Check sheet for the modelled part. Datum: model origin and axes. Units: mm. A direction names the side the tool comes from. Coordinates: 2 decimals unless noted, no trailing zeros. Write each loop counter-clockwise with the first axis right and the second up, starting at its lowest first coordinate (ties: lowest second). Pieces come first, ordered by that corner, then holes. Notation, with made-up numbers: M 1,39.25 L 7,39.25 A10 ccw 7,56.25 Z; hole C 22,84.25 d9. An arc over 180 degrees is marked long. Answer as CSV lines item,"result". Start each with the question number.
Q1. Sectioned sample at D-D, the plane z = 3.75. Record the cut outline in (x, y), then the cut area to 3 significant figures.
Q2. Mould release check, pull along X, two halves, no side actions. Record for faces 4 (the cylindrical face through (2.744, -3.517, 2.771)), 5 (the flat face through (-1.4, -4.5, -4.2)), 6 (the cylindrical face through (2.42, -4.36, 2.39)), 7 (the cylindrical face through (-2.42, -4.36, -2.39)): pulls with the +X half, pulls with the -X half, needs draft (parallel to the pull), parting line crosses it, or undercut.
Q3. Sectioned sample at B-B, the plane y = -3.3. Count the separate pieces of the cut face and the enclosed holes in it, then the cut area to 3 significant figures.
Q4. Sectioned sample at C-C, the plane z = 0. Record the cut outline in (x, y) (3 decimals).
Q5. Access from +Z, -Z, +X, -X, +Y, -Y to the whole of each face (thin tool, end or side, straight path). Record for faces 1 (the cylindrical face through (4.725, -4.192, 0.02)), 2 (the cylindrical face through (0, -4.3, 4.4)), 3 (the cylindrical face through (2.48, -2.96, 2.47)).
Q6. Depth check by flat-ended pin: pin 1 Ø0.6 at (x, y) = (-5, -4.5) entering from -Z; pin 2 Ø1.2 at (y, z) = (-4.5, 4.5) entering from -X; pin 3 Ø0.6 at (x, z) = (0.5, -4.5) entering from +Y. Enter the tip coordinate at first touch or a pass-through.
Q7. Sectioned sample at A-A, the plane x = 0. Record the cut outline in (y, z) (3 decimals).
Q8. Thickness scan on line 1 along Z through (x, y) = (-1, -3.95); line 2 along X through (y, z) = (-4.15, -3); line 3 along X through (y, z) = (-4.15, 2). Record the ranges inside material, lowest first. Write a range as from..to.
from build123d import *

# Parameters (mm, degrees)
SKETCH_1_R          = 3.4
EXTRUDE_1_DEPTH     = 1.1
EXTRUDE_START       = -0.362295
EXTRUDE_2_DEPTH     = 1.1
EXTRUDE_START_2     = -1.1
EXTRUDE_3_DEPTH     = 0.3
EXTRUDE_START_3     = 1.1
EXTRUDE_4_DEPTH     = 1.7
FILLET_2_R          = 0.5
FILLET_3_R          = 0.4
CUT_EXTRUDE_1_DEPTH = 8.685701009
FILLET_5_R          = 0.4


with BuildPart() as part:
    # 草图1 → 凸台-拉伸1 (new body)
    with BuildSketch(Plane.XZ.offset(4.897705057)):
        with BuildLine():
            Line((1.4, 4.38178046), (1.4, 3.640054945))
            ThreePointArc((1.4, 3.640054945), (2.757716447, 2.757716447), (3.640054945, 1.4))
            Line((3.640054945, 1.4), (4.38178046, 1.4))
            ThreePointArc((4.38178046, 1.4), (4.6, 0), (4.38178046, -1.4))
            Line((4.38178046, -1.4), (3.640054945, -1.4))
            ThreePointArc((3.640054945, -1.4), (2.757716447, -2.757716447), (1.4, -3.640054945))
            Line((1.4, -3.640054945), (1.4, -4.38178046))
            ThreePointArc((1.4, -4.38178046), (0, -4.6), (-1.4, -4.38178046))
            Line((-1.4, -4.38178046), (-1.4, -3.640054945))
            ThreePointArc((-1.4, -3.640054945), (-2.757716447, -2.757716447), (-3.640054945, -1.4))
            Line((-3.640054945, -1.4), (-4.38178046, -1.4))
            ThreePointArc((-4.38178046, -1.4), (-4.6, 0), (-4.38178046, 1.4))
            Line((-4.38178046, 1.4), (-3.640054945, 1.4))
            ThreePointArc((-3.640054945, 1.4), (-2.757716447, 2.757716447), (-1.4, 3.640054945))
            Line((-1.4, 3.640054945), (-1.4, 4.38178046))
            ThreePointArc((-1.4, 4.38178046), (0, 4.6), (1.4, 4.38178046))
        make_face()
        with Locations(Location((0, 0, 0), (0, 0, 270))):
            Circle(SKETCH_1_R, mode=Mode.SUBTRACT)
    extrude(amount=-EXTRUDE_1_DEPTH)

    # 草图2 → 凸台-拉伸2 (add)
    with BuildSketch(Plane.XZ.offset(4.16).offset(EXTRUDE_START)):
        with BuildLine():
            Line((4.276680956, 1.4), (4.512828935, 1.4))
            ThreePointArc((4.512828935, 1.4), (4.725, 0), (4.512828935, -1.4))
            Line((4.512828935, -1.4), (4.276680956, -1.4))
            ThreePointArc((4.276680956, -1.4), (4.5, 0), (4.276680956, 1.4))
        make_face()
        with BuildLine():
            Line((1.4, -4.276680956), (1.4, -4.512828935))
            ThreePointArc((1.4, -4.512828935), (0, -4.725), (-1.4, -4.512828935))
            Line((-1.4, -4.512828935), (-1.4, -4.276680956))
            ThreePointArc((-1.4, -4.276680956), (0, -4.5), (1.4, -4.276680956))
        make_face()
        with BuildLine():
            Line((-4.276680956, -1.4), (-4.512828935, -1.4))
            ThreePointArc((-4.512828935, -1.4), (-4.725, 0), (-4.512828935, 1.4))
            Line((-4.512828935, 1.4), (-4.276680956, 1.4))
            ThreePointArc((-4.276680956, 1.4), (-4.5, 0), (-4.276680956, -1.4))
        make_face()
        with BuildLine():
            Line((-1.4, 4.276680956), (-1.4, 4.512828935))
            ThreePointArc((-1.4, 4.512828935), (0, 4.725), (1.4, 4.512828935))
            Line((1.4, 4.512828935), (1.4, 4.276680956))
            ThreePointArc((1.4, 4.276680956), (0, 4.5), (-1.4, 4.276680956))
        make_face()
    extrude(amount=EXTRUDE_2_DEPTH)

    # 草图3 → 凸台-拉伸3 (add)
    with BuildSketch(Plane(origin=(0, -3.797705057, 0), x_dir=(-1, 0, 0), z_dir=(0, 1, 0)).offset(EXTRUDE_START_2)):
        with BuildLine():
            Line((4.276680956, 1.4), (5.111751168, 1.4))
            ThreePointArc((5.111751168, 1.4), (5.3, 0), (5.111751168, -1.4))
            Line((5.111751168, -1.4), (4.276680956, -1.4))
            ThreePointArc((4.276680956, -1.4), (4.5, 0), (4.276680956, 1.4))
        make_face()
        with BuildLine():
            Line((-1.4, -4.276680956), (-1.4, -5.111751168))
            ThreePointArc((-1.4, -5.111751168), (0, -5.3), (1.4, -5.111751168))
            Line((1.4, -5.111751168), (1.4, -4.276680956))
            ThreePointArc((1.4, -4.276680956), (0, -4.5), (-1.4, -4.276680956))
        make_face()
        with BuildLine():
            Line((-4.276680956, 1.4), (-5.111751168, 1.4))
            ThreePointArc((-5.111751168, 1.4), (-5.3, 0), (-5.111751168, -1.4))
            Line((-5.111751168, -1.4), (-4.276680956, -1.4))
            ThreePointArc((-4.276680956, -1.4), (-4.5, 0), (-4.276680956, 1.4))
        make_face()
        with BuildLine():
            Line((1.4, 4.276680956), (1.4, 5.111751168))
            ThreePointArc((1.4, 5.111751168), (0, 5.3), (-1.4, 5.111751168))
            Line((-1.4, 5.111751168), (-1.4, 4.276680956))
            ThreePointArc((-1.4, 4.276680956), (0, 4.5), (1.4, 4.276680956))
        make_face()
    extrude(amount=EXTRUDE_3_DEPTH)

    # 草图4 → 凸台-拉伸4 (add)
    with BuildSketch(Plane(origin=(0, -4.897705057, 0), x_dir=(-1, 0, 0), z_dir=(0, 1, 0)).offset(EXTRUDE_START_3)):
        with BuildLine():
            Line((1.55, 3.578756767), (1.55, 3.138072657))
            ThreePointArc((1.55, 3.138072657), (2.474873734, 2.474873734), (3.138072657, 1.55))
            Line((3.138072657, 1.55), (3.578756767, 1.55))
            ThreePointArc((3.578756767, 1.55), (2.757716447, 2.757716447), (1.55, 3.578756767))
        make_face()
        with BuildLine():
            Line((1.55, -3.138072657), (1.55, -3.578756767))
            ThreePointArc((1.55, -3.578756767), (2.757716447, -2.757716447), (3.578756767, -1.55))
            Line((3.578756767, -1.55), (3.138072657, -1.55))
            ThreePointArc((3.138072657, -1.55), (2.474873734, -2.474873734), (1.55, -3.138072657))
        make_face()
        with BuildLine():
            Line((-3.138072657, -1.55), (-3.578756767, -1.55))
            ThreePointArc((-3.578756767, -1.55), (-2.757716447, -2.757716447), (-1.55, -3.578756767))
            Line((-1.55, -3.578756767), (-1.55, -3.138072657))
            ThreePointArc((-1.55, -3.138072657), (-2.474873734, -2.474873734), (-3.138072657, -1.55))
        make_face()
        with BuildLine():
            Line((-1.55, 3.138072657), (-1.55, 3.578756767))
            ThreePointArc((-1.55, 3.578756767), (-2.757716447, 2.757716447), (-3.578756767, 1.55))
            Line((-3.578756767, 1.55), (-3.138072657, 1.55))
            ThreePointArc((-3.138072657, 1.55), (-2.474873734, 2.474873734), (-1.55, 3.138072657))
        make_face()
    extrude(amount=EXTRUDE_4_DEPTH)

    # 圆角2
    fillet_2_edges = [part.edges().sort_by_distance(p)[0] for p in [
        (1.55, -2.947705057, 3.138072657),
        (3.138072657, -2.947705057, 1.55),
        (3.138072657, -2.947705057, -1.55),
        (1.55, -2.947705057, -3.138072657),
        (-1.55, -2.947705057, -3.138072657),
        (-3.138072657, -2.947705057, -1.55),
        (-3.138072657, -2.947705057, 1.55),
        (-1.55, -2.947705057, 3.138072657),
    ]]
    fillet(fillet_2_edges, radius=FILLET_2_R)

    # 圆角3
    fillet_3_edges = [part.edges().sort_by_distance(p)[0] for p in [
        (-3.640054945, -4.347705057, 1.4),
        (-3.640054945, -4.347705057, -1.4),
        (-1.4, -4.347705057, -3.640054945),
        (1.4, -4.347705057, -3.640054945),
        (3.640054945, -4.347705057, -1.4),
        (3.640054945, -4.347705057, 1.4),
        (1.4, -4.347705057, 3.640054945),
        (-1.4, -4.347705057, 3.640054945),
    ]]
    fillet(fillet_3_edges, radius=FILLET_3_R)

    # 草图5 → 切除-拉伸1 (cut, through all)
    with BuildSketch(Plane(origin=(0, -3.797705057, 0), x_dir=(-1, 0, 0), z_dir=(0, 1, 0))):
        with BuildLine():
            Line((4.306971093, 0.9), (2.740001738, 0.9))
            Line((2.740001738, 0.9), (2.740001738, -0.9))
            Line((2.740001738, -0.9), (4.306971093, -0.9))
            ThreePointArc((4.306971093, -0.9), (4.4, 0), (4.306971093, 0.9))
        make_face()
        with BuildLine():
            Line((0.9, -4.306971093), (0.9, -2.740001738))
            Line((0.9, -2.740001738), (-0.9, -2.740001738))
            Line((-0.9, -2.740001738), (-0.9, -4.306971093))
            ThreePointArc((-0.9, -4.306971093), (0, -4.4), (0.9, -4.306971093))
        make_face()
        with BuildLine():
            Line((-4.306971093, -0.9), (-2.740001738, -0.9))
            Line((-2.740001738, -0.9), (-2.740001738, 0.9))
            Line((-2.740001738, 0.9), (-4.306971093, 0.9))
            ThreePointArc((-4.306971093, 0.9), (-4.4, 0), (-4.306971093, -0.9))
        make_face()
        with BuildLine():
            Line((-0.9, 4.306971093), (-0.9, 2.740001738))
            Line((-0.9, 2.740001738), (0.9, 2.740001738))
            Line((0.9, 2.740001738), (0.9, 4.306971093))
            ThreePointArc((0.9, 4.306971093), (0, 4.4), (-0.9, 4.306971093))
        make_face()
    extrude(amount=-CUT_EXTRUDE_1_DEPTH, mode=Mode.SUBTRACT)

    # 圆角5
    fillet_5_edges = [part.edges().sort_by_distance(p)[0] for p in [
        (0.9, -4.347705057, 3.278719262),
        (-0.9, -4.347705057, 3.278719262),
        (3.278719262, -4.347705057, -0.9),
        (3.278719262, -4.347705057, 0.9),
        (-0.9, -4.347705057, -3.278719262),
        (0.9, -4.347705057, -3.278719262),
        (-3.278719262, -4.347705057, 0.9),
        (-3.278719262, -4.347705057, -0.9),
        (-4.306971093, -4.347705057, -0.9),
        (-4.306971093, -4.347705057, 0.9),
        (0.9, -4.347705057, -4.306971093),
        (-0.9, -4.347705057, -4.306971093),
        (4.306971093, -4.347705057, 0.9),
        (4.306971093, -4.347705057, -0.9),
        (-0.9, -4.347705057, 4.306971093),
        (0.9, -4.347705057, 4.306971093),
    ]]
    fillet(fillet_5_edges, radius=FILLET_5_R)


solid = part.part
Output:
1,outline,"M -1.43,-4.9 L -0.9,-4.9 L -0.9,-3.8 L -1.43,-3.8 Z; M 0.9,-4.9 L 1.43,-4.9 L 1.43,-3.8 L 0.9,-3.8 Z"
1,area,"1.17 mm^2"
2,face 4,"pulls with the +X half"
2,face 5,"pulls with the -X half"
2,face 6,"undercut"
2,face 7,"undercut"
3,separate pieces,"4"
3,enclosed holes,"0"
3,area,"4.07 mm^2"
4,outline,"M -5.3,-4.898 L -4.4,-4.898 L -4.4,-3.798 L -4.725,-3.798 L -4.725,-4.598 L -5.3,-4.598 Z; M 4.4,-4.898 L 5.3,-4.898 L 5.3,-4.598 L 4.725,-4.598 L 4.725,-3.798 L 4.4,-3.798 Z"
5,face 1,"+X, +Y"
5,face 2,"+Y, -Y"
5,face 3,"+Y"
6,pin 1,"stops at z = -1.4"
6,pin 2,"stops at x = -1.4"
6,pin 3,"stops at y = -3.8"
7,outline,"M -4.898,-5.3 L -4.598,-5.3 L -4.598,-4.725 L -3.798,-4.725 L -3.798,-4.4 L -4.898,-4.4 Z; M -4.898,4.4 L -3.798,4.4 L -3.798,4.725 L -4.598,4.725 L -4.598,5.3 L -4.898,5.3 Z"
8,line 1,"z = -4.62..-3.31, 3.31..4.62"
8,line 2,"x = -2.49..-1.6, 1.6..2.49"
8,line 3,"x = -3.35..-2.75, 2.75..3.35"
